For this review, take the finished solid that the model builds, in its own axes (mm). Give positions to 0.01 mm unless a question says otherwise; leave off trailing zeros. Loops run counter-clockwise (first coordinate to the right, second up) from the corner with the lowest first, then second, coordinate; pieces in that order, holes last.
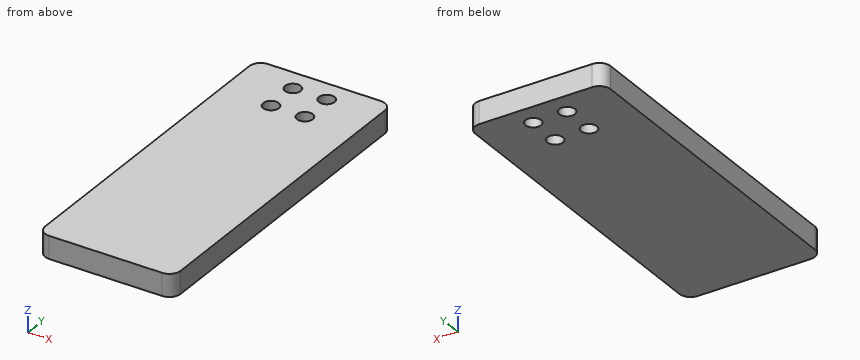
```python
from build123d import *

# Parameters (mm, degrees)
IZIM1_W               = 60
IZIM1_H               = 150
TABAN_FLAN_1_DEPTH    = 10
IZIM6_R               = 3.5
KES_EKSTR_ZYON1_DEPTH = 26
RADYUS1_R             = 5


# Sheet-metal steps are written as plain solids
with BuildPart() as part:
    # Çizim1 → Taban-Flanş1 (new body)
    with BuildSketch(Plane.XY):
        Rectangle(IZIM1_W, IZIM1_H)
    extrude(amount=-TABAN_FLAN_1_DEPTH)

    # Çizim6 → Kes-Ekstrüzyon1 (cut)
    with BuildSketch(Plane.XY):
        with Locations((7.5, 65)):
            Circle(IZIM6_R)
        with Locations((-7.5, 65)):
            Circle(IZIM6_R)
        with Locations((7.5, 50)):
            Circle(IZIM6_R)
        with Locations((-7.5, 50)):
            Circle(IZIM6_R)
    extrude(amount=-KES_EKSTR_ZYON1_DEPTH, mode=Mode.SUBTRACT)

    # Radyus1
    radyus1_edges = [part.edges().sort_by_distance(p)[0] for p in [
        (30, -75, -5),
        (-30, -75, -5),
        (-30, 75, -5),
        (30, 75, -5),
    ]]
    fillet(radyus1_edges, radius=RADYUS1_R)


solid = part.part
```
Q1. Consider section B-B on x = 7.5. Give the boundary of the cut face in (y, z).
Answers:
outline: (-75, -10) - (46.5, -10) - (46.5, 0) - (-75, 0) - close; (53.5, -10) - (61.5, -10) - (61.5, 0) - (53.5, 0) - close; (68.5, -10) - (75, -10) - (75, 0) - (68.5, 0) - close
Q2. For probe 1 along Y at (x, z) = (-7.5, -7.75); probe 2 along Y at (x, z) = (5.5, -7.5); probe 3 along Y at (x, z) = (26.5, -3.75), list the stretches that pass through material, from the lowest coordinate up.
Answers:
probe 1: y = -75 to 46.5, 53.5 to 61.5, 68.5 to 75
probe 2: y = -75 to 47.13, 52.87 to 62.13, 67.87 to 75
probe 3: y = -74.77 to 74.77
Q3. Consider section A-A on y = 65. Give the boundary of the cut face in (x, z).
Answers:
outline: (-30, -10) - (-11, -10) - (-11, 0) - (-30, 0) - close; (-4, -10) - (4, -10) - (4, 0) - (-4, 0) - close; (11, -10) - (30, -10) - (30, 0) - (11, 0) - close
Q4. Consider section C-C on z = -6.25. Give the boundary of the cut face in (x, y), plus the area to 3 significant figures.
Answers:
outline: (-30, -70) arc R5 ccw to (-25, -75) - (25, -75) arc R5 ccw to (30, -70) - (30, 70) arc R5 ccw to (25, 75) - (-25, 75) arc R5 ccw to (-30, 70) - close; hole circle Ø7 at (-7.5, 50); hole circle Ø7 at (-7.5, 65); hole circle Ø7 at (7.5, 50); hole circle Ø7 at (7.5, 65)
area: 8,820 mm2
